Build history of the part. All positions in model axes, mm. A direction names the side the tool comes from. Round coordinates to 2 decimals unless told otherwise and drop trailing zeros. Order: outer loops, then holes, each group sorted by start corner. A loop starts at its lowest first (then second) coordinate and runs counter-clockwise, first axis right, second up. Notation, with made-up numbers: M 0,22 L 23,22 A12 ccw 23,34 Z; hole C -7,64 d3. An arc over 180 degrees is marked long. One line per question, with ' | ' between items. Start each with the question number.
from build123d import *

# Parameters (mm, degrees)
SKETCH1_W           = 75
SKETCH1_H           = 300
BOSS_EXTRUDE1_DEPTH = 75
CUT_EXTRUDE1_START  = -75
CUT_EXTRUDE1_DEPTH  = 45


with BuildPart() as part:
    # Sketch1 → Boss-Extrude1 (new, symmetric)
    with BuildSketch(Plane.XY):
        with Locations((37.5, 150)):
            Rectangle(SKETCH1_W, SKETCH1_H)
    extrude(amount=BOSS_EXTRUDE1_DEPTH, both=True)

    # Sketch2 → Cut-Extrude1 (cut, symmetric)
    with BuildSketch(Plane.XY.offset(75).offset(CUT_EXTRUDE1_START)):
        Polygon((75, 290), (37.5, 252.5), (75, 215), align=None)
    extrude(amount=CUT_EXTRUDE1_DEPTH, both=True, mode=Mode.SUBTRACT)


solid = part.part
Item 1: Wall check: line 1 along Z through (x, y) = (66.5, 233.5); line 2 along Y through (x, z) = (64, -7.5); line 3 along Y through (x, z) = (64.5, -40). Give the ranges that are in metal, low to high. Write a range as [from, to].
Item 2: Tool access for faces 1 (the face through (57, 272, 1)), 2 (the face through (37, 152, -75)): list every direction of +Z, -Z, +X, -X, +Y, -Y with a clear straight run to the whole face (end or side of a thin tool).
Item 3: Cut at B-B on y = 233.5. Write the cut outline in (x, z).
Item 4: Two-plate mould, pull along Y, no slides. Class faces 3 (the face through (37, 0, 1)), 4 (the face through (60, 253, -45)), 5 (the face through (0, 148, 1)): +Y half, -Y half, draft (parallel to the pull), parting line (faces both ways), or undercut.
Item 5: Cut at D-D on x = 42. Write the cut outline in (y, z).
Item 6: Cut at C-C on z = 24. Write the cut outline in (x, y).
Item 7: Cut at A-A on x = 57. Write the cut outline in (y, z), then the cut area to 3 significant figures.
Results found:
1) line 1: z = [-75, -45], [45, 75] | line 2: y = [0, 226], [279, 300] | line 3: y = [0, 225.5], [279.5, 300]
2) face 1: +X | face 2: -Z, +X, -X, +Y, -Y
3) outline: M 0,-75 L 75,-75 L 75,-45 L 56.5,-45 L 56.5,45 L 75,45 L 75,75 L 0,75 Z
4) face 3: -Y half | face 4: undercut | face 5: draft
5) outline: M 0,-75 L 300,-75 L 300,75 L 0,75 Z; hole M 248,-45 L 257,-45 L 257,45 L 248,45 Z
6) outline: M 0,0 L 75,0 L 75,215 L 37.5,252.5 L 75,290 L 75,300 L 0,300 Z
7) outline: M 0,-75 L 300,-75 L 300,75 L 0,75 Z; hole M 233,-45 L 272,-45 L 272,45 L 233,45 Z | area: 41,500 mm^2
